The model under review builds one solid part; all positions refer to its coordinate system, in mm. Face numbers are marked on the shaded views. A direction names the side the tool comes from. Coordinates: 2 decimals unless noted, no trailing zeros. Order: outer loops, then holes, each group sorted by start corner. A loop starts at its lowest first (then second) coordinate and runs counter-clockwise, first axis right, second up. Notation, with made-up numbers: M 19.5,62 L 35.5,62 A22 cw 35.5,73 Z; hole C -6,54 d9. An arc over 180 degrees is marked long. Answer as CSV lines item,"result". Start each with the question number.
Q1. Consider section B-B on x = 8. Write out the cut boundary in (y, z).
Q2. The part is to be moulded in two halves that separate along Z. For the marked faces 3, 4 and 5, say which applies: +Z half, -Z half, draft (parallel to the pull), parting line (faces both ways), or undercut.
Q3. Consider section A-A on z = 0. Write out the cut boundary in (x, y), and give its area (3 significant figures).
Q4. Consider section C-C on z = 8. Write out the cut boundary in (x, y), and give its area (3 significant figures).
Q5. Machinability: for the marked faces 1 and 2, which of the approach directions +Z, -Z, +X, -X, +Y, -Y give a long, thin tool a straight path to every point of the face, cutting with its end or side? Answer none if there is none.
Q6. Consider section D-D on y = 35. Write out the cut boundary in (x, z) (3 decimals), and give its area (3 significant figures).
Q7. For P1, Ø1, axis at x = 0, z = -6.5, coming from the +Y side; P2, Ø1.6, axis at x = -22.5, z = 27, coming from the -Y side; P3, Ø1.2, axis at x = -7, z = 0, coming from the -Y side; P4, Ø1, axis at x = -17, y = 36, coming from the -Z side, all flat-tipped, find the tip position at first contact; note any pin that passes through.
Q8. Wall thickness on L1, parallel to Y at x = -23, z = 26.65 (3 decimals); L2, parallel to Y at x = -23, z = 28; L3, parallel to X at y = 2, z = 21: over which ranges is each line inside the solid? List them lowest first. Write a range as [from, to].
from build123d import *

# Parameters (mm, degrees)
SKETCH2_W           = 25
SKETCH2_H           = 41
BOSS_EXTRUDE1_DEPTH = 5
SKETCH4_W           = 25
SKETCH4_H           = 41
BOSS_EXTRUDE2_DEPTH = 5
SKETCH5_W           = 18
SKETCH5_H           = 5
BOSS_EXTRUDE3_DEPTH = 41
SKETCH6_R           = 2.075
CUT_EXTRUDE1_DEPTH  = 5
SKETCH11_R          = 2.075
SKETCH11_R_2        = 1.7
BOSS_EXTRUDE5_DEPTH = 1.5
SKETCH12_W          = 18
SKETCH12_H          = 6
BOSS_EXTRUDE6_DEPTH = 5
FILLET5_R           = 2
SKETCH13_R          = 2
CUT_EXTRUDE2_DEPTH  = 1.5
CUT_EXTRUDE7_DEPTH  = 6.5


with BuildPart() as part:
    # Sketch2 → Boss-Extrude1 (new body)
    with BuildSketch(Plane(origin=(0, 0, 0), x_dir=(1, 0, 0), z_dir=(0, 1, 0))):
        with Locations((0, -3.5)):
            Rectangle(SKETCH2_W, SKETCH2_H)
        with BuildLine():
            ThreePointArc((0, -6.95), (-1.05, -8), (0, -9.05))
            ThreePointArc((0, -9.05), (1.05, -8), (0, -6.95))
        make_face(mode=Mode.SUBTRACT)
        with BuildLine():
            ThreePointArc((-8, 1.05), (-9.05, 0), (-8, -1.05))
            ThreePointArc((-8, -1.05), (-6.95, 0), (-8, 1.05))
        make_face(mode=Mode.SUBTRACT)
        with BuildLine():
            ThreePointArc((8, 1.05), (6.95, 0), (8, -1.05))
            ThreePointArc((8, -1.05), (9.05, 0), (8, 1.05))
        make_face(mode=Mode.SUBTRACT)
        with BuildLine():
            ThreePointArc((0, 6.95), (1.05, 8), (0, 9.05))
            ThreePointArc((0, 9.05), (-1.05, 8), (0, 6.95))
        make_face(mode=Mode.SUBTRACT)
    extrude(amount=BOSS_EXTRUDE1_DEPTH)

    # Sketch4 → Boss-Extrude2 (add)
    with BuildSketch(Plane.XY.offset(24)):
        with Locations((0, 20.5)):
            Rectangle(SKETCH4_W, SKETCH4_H)
    extrude(amount=BOSS_EXTRUDE2_DEPTH)

    # Sketch5 → Boss-Extrude3 (add)
    with BuildSketch(Plane.XZ):
        with Locations((-21.5, 26.5)):
            Rectangle(SKETCH5_W, SKETCH5_H)
    extrude(amount=-BOSS_EXTRUDE3_DEPTH)

    # Sketch6 → Cut-Extrude1 (cut)
    with BuildSketch(Plane.XY.offset(29)):
        with Locations((-23, 13)):
            Circle(SKETCH6_R)
        with Locations((-23, 35)):
            Circle(SKETCH6_R)
    extrude(amount=-CUT_EXTRUDE1_DEPTH, mode=Mode.SUBTRACT)

    # Sketch11 → Boss-Extrude5 (add)
    with BuildSketch(Plane.XY.offset(29)):
        with Locations((-23, 13)):
            Circle(SKETCH11_R)
        with Locations((-23, 13)):
            Circle(SKETCH11_R_2, mode=Mode.SUBTRACT)
        with Locations((-23, 35)):
            Circle(SKETCH11_R)
        with Locations((-23, 35)):
            Circle(SKETCH11_R_2, mode=Mode.SUBTRACT)
    extrude(amount=-BOSS_EXTRUDE5_DEPTH)

    # Sketch12 → Boss-Extrude6 (add)
    with BuildSketch(Plane.XZ):
        with Locations((-21.5, 21)):
            Rectangle(SKETCH12_W, SKETCH12_H)
    extrude(amount=-BOSS_EXTRUDE6_DEPTH)

    # Fillet5
    fillet5_edges = [part.edges().sort_by_distance(p)[0] for p in [
        (-30.5, 2.5, 18),
    ]]
    fillet(fillet5_edges, radius=FILLET5_R)

    # Sketch13 → Cut-Extrude2 (cut)
    with BuildSketch(Plane(origin=(0, 0, 0), x_dir=(-1, 0, 0), z_dir=(0, -1, 0))):
        with Locations((0, -8)):
            Circle(SKETCH13_R)
        with Locations((8, 0)):
            Circle(SKETCH13_R)
        with Locations((0, 8)):
            Circle(SKETCH13_R)
        with Locations((-8, 0)):
            Circle(SKETCH13_R)
    extrude(amount=-CUT_EXTRUDE2_DEPTH, mode=Mode.SUBTRACT)

    # Sketch15 → Cut-Extrude7 (cut)
    with BuildSketch(Plane.XZ):
        with BuildLine():
            Line((-21.744637892, 29), (-21.744637892, 18))
            Line((-21.744637892, 18), (-21.794637892, 18))
            Line((-21.794637892, 18), (-22.424637892, 18))
            Line((-22.424637892, 18), (-22.424637892, 18.259824575))
            ThreePointArc((-22.424637892, 18.259824575), (-22.46186648, 18.358731646), (-22.555072675, 18.408543109))
            ThreePointArc((-22.555072675, 18.408543109), (-22.712700046, 18.442388286), (-22.862840139, 18.501123596))
            ThreePointArc((-22.862840139, 18.501123596), (-23.174637892, 19), (-22.862840139, 19.498876404))
            ThreePointArc((-22.862840139, 19.498876404), (-22.712700046, 19.557611714), (-22.555072675, 19.591456891))
            ThreePointArc((-22.555072675, 19.591456891), (-22.46186648, 19.641268354), (-22.424637892, 19.740175425))
            Line((-22.424637892, 19.740175425), (-22.424637892, 20.259824575))
            ThreePointArc((-22.424637892, 20.259824575), (-22.46186648, 20.358731646), (-22.555072675, 20.408543109))
            ThreePointArc((-22.555072675, 20.408543109), (-22.712700046, 20.442388286), (-22.862840139, 20.501123596))
            ThreePointArc((-22.862840139, 20.501123596), (-23.174637892, 21), (-22.862840139, 21.498876404))
            ThreePointArc((-22.862840139, 21.498876404), (-22.712700046, 21.557611714), (-22.555072675, 21.591456891))
            ThreePointArc((-22.555072675, 21.591456891), (-22.46186648, 21.641268354), (-22.424637892, 21.740175425))
            Line((-22.424637892, 21.740175425), (-22.424637892, 22.259824575))
            ThreePointArc((-22.424637892, 22.259824575), (-22.46186648, 22.358731646), (-22.555072675, 22.408543109))
            ThreePointArc((-22.555072675, 22.408543109), (-22.712700046, 22.442388286), (-22.862840139, 22.501123596))
            ThreePointArc((-22.862840139, 22.501123596), (-23.174637892, 23), (-22.862840139, 23.498876404))
            ThreePointArc((-22.862840139, 23.498876404), (-22.712700046, 23.557611714), (-22.555072675, 23.591456891))
            ThreePointArc((-22.555072675, 23.591456891), (-22.46186648, 23.641268354), (-22.424637892, 23.740175425))
            Line((-22.424637892, 23.740175425), (-22.424637892, 24.259824575))
            ThreePointArc((-22.424637892, 24.259824575), (-22.46186648, 24.358731646), (-22.555072675, 24.408543109))
            ThreePointArc((-22.555072675, 24.408543109), (-22.712700046, 24.442388286), (-22.862840139, 24.501123596))
            ThreePointArc((-22.862840139, 24.501123596), (-23.174637892, 25), (-22.862840139, 25.498876404))
            ThreePointArc((-22.862840139, 25.498876404), (-22.712700046, 25.557611714), (-22.555072675, 25.591456891))
            ThreePointArc((-22.555072675, 25.591456891), (-22.46186648, 25.641268354), (-22.424637892, 25.740175425))
            Line((-22.424637892, 25.740175425), (-22.424637892, 26.259824575))
            ThreePointArc((-22.424637892, 26.259824575), (-22.46186648, 26.358731646), (-22.555072675, 26.408543109))
            ThreePointArc((-22.555072675, 26.408543109), (-22.712700046, 26.442388286), (-22.862840139, 26.501123596))
            ThreePointArc((-22.862840139, 26.501123596), (-23.174637892, 27), (-22.862840139, 27.498876404))
            ThreePointArc((-22.862840139, 27.498876404), (-22.712700046, 27.557611714), (-22.555072675, 27.591456891))
            ThreePointArc((-22.555072675, 27.591456891), (-22.46186648, 27.641268354), (-22.424637892, 27.740175425))
            Line((-22.424637892, 27.740175425), (-22.424637892, 28.259824575))
            ThreePointArc((-22.424637892, 28.259824575), (-22.46186648, 28.358731646), (-22.555072675, 28.408543109))
            ThreePointArc((-22.555072675, 28.408543109), (-22.712700046, 28.442388286), (-22.862840139, 28.501123596))
            ThreePointArc((-22.862840139, 28.501123596), (-23.090276951, 28.705850588), (-23.174637892, 29))
            Line((-23.174637892, 29), (-21.794637892, 29))
            Line((-21.794637892, 29), (-21.744637892, 29))
        make_face()
    extrude(amount=-CUT_EXTRUDE7_DEPTH, mode=Mode.SUBTRACT)


solid = part.part
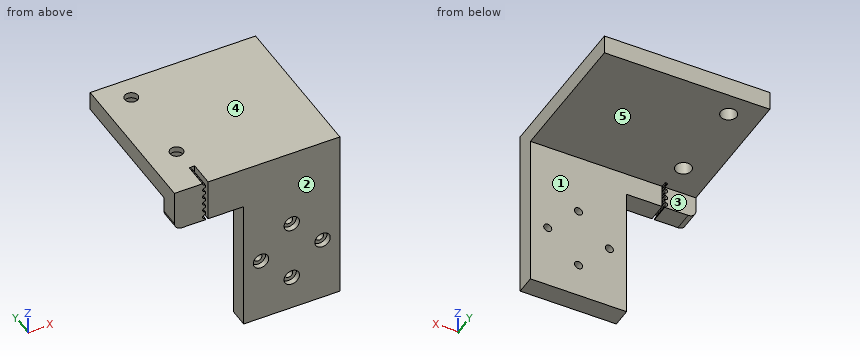
Evaluation:
1,outline,"M 0,-17 L 5,-17 L 5,-1.05 L 1.5,-1.05 L 1.5,-2 L 0,-2 Z; M 0,2 L 1.5,2 L 1.5,1.05 L 5,1.05 L 5,24 L 41,24 L 41,29 L 0,29 Z"
2,face 3,"draft"
2,face 4,"+Z half"
2,face 5,"-Z half"
3,outline,"M -12.5,0 L -10,0 L -10,1.5 L -9.05,1.5 L -9.05,5 L -12.5,5 Z; M -6.95,1.5 L -6,1.5 L -6,0 L 6,0 L 6,1.5 L 6.95,1.5 L 6.95,5 L -6.95,5 Z; M 9.05,1.5 L 10,1.5 L 10,0 L 12.5,0 L 12.5,5 L 9.05,5 Z"
3,area,"98.3 mm²"
4,outline,"M -12.5,0 L -2,0 L -2,1.5 L -1.05,1.5 L -1.05,5 L -12.5,5 Z; M 1.05,1.5 L 2,1.5 L 2,0 L 12.5,0 L 12.5,5 L 1.05,5 Z"
4,area,"112 mm²"
5,face 1,"-Z, +X, -X, +Y"
5,face 2,"+Z, -Z, +X, -X, -Y"
6,outline,"M -30.5,24 L -25.075,24 L -25.075,27.5 L -24.7,27.5 L -24.7,29 L -30.5,29 Z; M -21.3,27.5 L -20.925,27.5 L -20.925,24 L 12.5,24 L 12.5,29 L -21.3,29 Z"
6,area,"195 mm²"
7,P1,"stops at y = 5"
7,P2,"stops at y = 0"
7,P3,"stops at y = 1.5"
7,P4,"stops at z = 24"
8,L1,"y = [6.5, 10.925], [15.075, 32.925], [37.075, 41]"
8,L2,"y = [0, 11.3], [14.7, 33.3], [36.7, 41]"
8,L3,"x = [-30.5, -23.17], [-21.74, 12.5]"
